For this review, use the dimensioned drawing (mm, ordinates from the lowest corner) and the shaded views. Round coordinates to 2 decimals unless told otherwise and drop trailing zeros. Order: outer loops, then holes, each group sorted by start corner. A loop starts at its lowest first (then second) coordinate and runs counter-clockwise, first axis right, second up. Notation, with made-up numbers: M 79.5,12 L 131.5,12 A15 ccw 131.5,24 Z; hole C -20,44.25 d5. An arc over 180 degrees is marked long. Put each result on its own line as item: value.
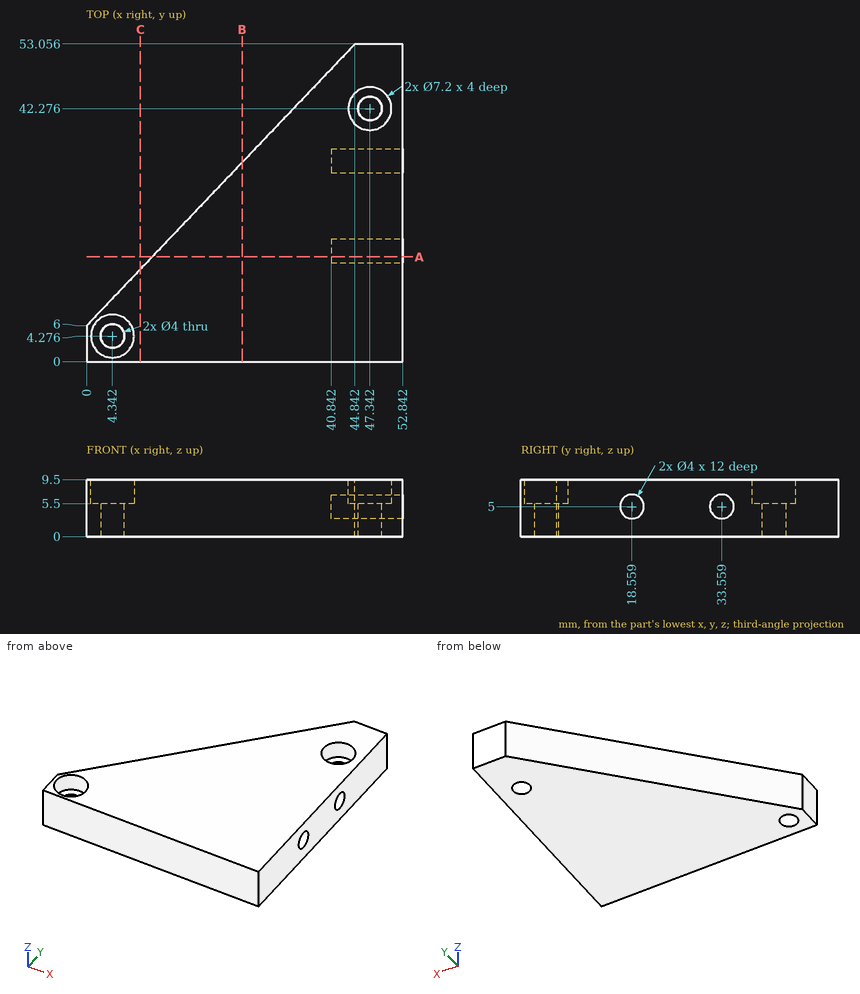
(1) Add section A-A on y = 17.5. Give the boundary of the cut face in (x, z).
A:
outline: M 10.96,0 L 52.84,0 L 52.84,3.3 L 40.84,3.3 L 40.84,6.7 L 52.84,6.7 L 52.84,9.5 L 10.96,9.5 Z
(2) Add section B-B on x = 26. Give the boundary of the cut face in (y, z), then the cut area to 3 significant figures.
A:
outline: M 0,0 L 33.28,0 L 33.28,9.5 L 0,9.5 Z
area: 316 mm2
(3) To check wall thickness, follow L1, parallel to Y at x = 41, z = 5.5 (1 decimal); L2, parallel to X at y = 4, z = 8.25; L3, parallel to X at y = 41.5, z = 0.5 (1 decimal). State the ranges of each line that lie inside material, in increasing order.
A:
L1: y = 0 to 16.6, 20.5 to 31.6, 35.5 to 49
L2: x = 0 to 0.75, 7.93 to 52.84
L3: x = 33.8 to 45.5, 49.2 to 52.8
(4) Add section C-C on x = 9. Give the boundary of the cut face in (y, z) (1 decimal), then the cut area to 3 significant figures.
A:
outline: M 0,0 L 15.4,0 L 15.4,9.5 L 0,9.5 Z
area: 147 mm2
(5) Insertion check: pin 1 Ø4 at (y, z) = (20, 4) entering from -X (1 decimal); pin 2 Ø4.5 at (x, y) = (47.34, 42.28) entering from +Z; pin 3 Ø2.5 at (y, z) = (33.56, 5) entering from -X. Each pin has a flat end and moves straight along its axis. Give the tip position at first contact, or say it passes through.
A:
pin 1: stops at x = 11.4
pin 2: stops at z = 5.5
pin 3: stops at x = 25.07
